Autodesk Inventor part; units mm, degrees
ref_plane "作業平面6" through (17, 0, 0) normal (1, 0, 0) x (0, 1, 0)
ref_plane "作業平面7" through (-17, 0, 0) normal (1, 0, 0) x (0, 1, 0)
ref_plane "作業平面8" through (0, 17, 0) normal (0, 1, 0) x (-1, 0, 0)
sketch "スケッチ1" plane through (0, 0, 0) normal (0, 0, 1) x (1, 0, 0)
  circle A0 centre (0, 0) radius 17
  circle A1 centre (0, 0) radius 11.5
  dimension "d0" = 34
  dimension "d1" = 23
extrude "押し出し1" add sketch "スケッチ1" against normal blind 40
sketch "スケッチ3" plane through (0, 0, 0) normal (0, 0, 1) x (1, 0, 0)
  circle A0 centre (0, 0) radius 15
  dimension "d8" = 30
extrude "押し出し3" cut sketch "スケッチ3" against normal blind 28
ref_plane "作業平面6" through (17, 0, 0) normal (1, 0, 0) x (0, 1, 0)
ref_plane "作業平面7" through (-17, 0, 0) normal (1, 0, 0) x (0, 1, 0)
sketch "スケッチ14" plane through (17, 0, 0) normal (1, 0, 0) x (0, 1, 0)
  point P0 (0, 0)
sketch "スケッチ15" plane through (17, 0, 0) normal (1, 0, 0) x (0, 1, 0)
  circle A0 centre (0, -5) radius 1.15
  point P0 (0, 0)
  dimension "d54" = 2.3
  dimension "d55" = 5
ref_plane "作業平面8" through (0, 17, 0) normal (0, 1, 0) x (-1, 0, 0)
ref_plane "作業平面9" through (0, -17, 0) normal (0, 1, 0) x (-1, 0, 0)
sketch "スケッチ16" plane through (0, 17, 0) normal (0, 1, 0) x (-1, 0, 0)
  circle A0 centre (0, -5) radius 1.15
  point P0 (0, 0)
  dimension "d58" = 2.3
  dimension "d59" = 5
extrude "押し出し13" cut sketch "スケッチ15" against normal through all
extrude "押し出し14" cut sketch "スケッチ16" against normal blind 5
sketch "スケッチ19" plane through (17, 0, 0) normal (1, 0, 0) x (0, 1, 0)
  circle A0 centre (0, -5) radius 2.1
  line L0 (17, 0) -> (-17, 0)
  point P0 (0, 0)
  dimension "d64" = 4.2
  dimension "d65" = 5
extrude "押し出し15" cut sketch "スケッチ19" against normal blind 1
sketch "スケッチ20" plane through (0, 17, 0) normal (0, 1, 0) x (-1, 0, 0)
  circle A0 centre (0, -5) radius 2.1
  line L0 (17, 0) -> (-17, 0)
  point P0 (0, 0)
  dimension "d68" = 4.2
  dimension "d69" = 5
extrude "押し出し16" cut sketch "スケッチ20" against normal blind 1
sketch "スケッチ21" plane through (-17, 0, 0) normal (1, 0, 0) x (0, 1, 0)
  circle A0 centre (0, -5) radius 2.1
  line L0 (17, 0) -> (-17, 0)
  point P0 (0, 0)
  dimension "d72" = 4.2
  dimension "d73" = 5
extrude "押し出し17" cut sketch "スケッチ21" along normal blind 1
sketch "スケッチ22" plane through (0, -17, 0) normal (0, 1, 0) x (-1, 0, 0)
  point P0 (0, 0)
sketch "スケッチ24" plane through (0, 0, -40) normal (0, 0, -1) x (-1, 0, 0)
  circle A0 centre (0, 0) radius 17
  circle A1 centre (0, 0) radius 13.4
  dimension "d80" = 26.8
  dimension "d83" = 34
extrude "押し出し19" cut sketch "スケッチ24" against normal blind 10
equation "\"BendRadius\" = Thickness"
equation "\"BendReliefWidth\" = Thickness"
equation "\"BendReliefDepth\" = 0.5 * Thickness"
equation "\"CornerReliefSize\" = 4 * Thickness"
equation "\"MinimumRemnant\" = 2 * Thickness"
equation "\"TransitionRadius\" = BendRadius"
equation "\"JacobiRadiusSize\" = BendRadius"
equation "\"GapSize\" = Thickness"
properties part number "B_pipe_adapter_1" material "ステンレス鋼 440C"
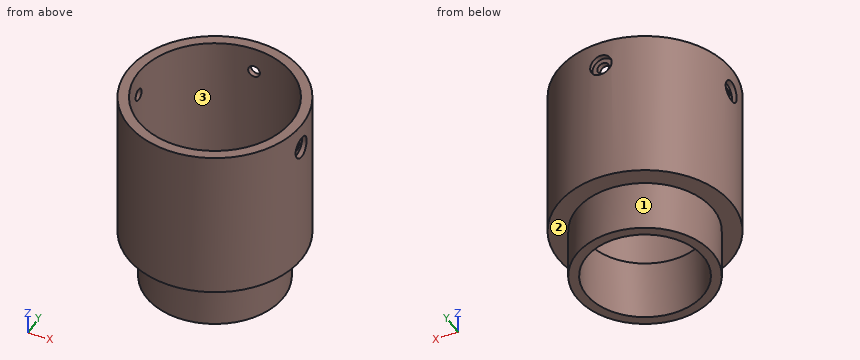
Here's how the part is built. I have some questions about the finished solid (model axes, mm). Face numbers are marked on the shaded views. Coordinates: 2 decimals unless noted, no trailing zeros. Loops run counter-clockwise (first coordinate to the right, second up) from the corner with the lowest first, then second, coordinate; pieces in that order, holes last. Notation, with made-up numbers: (88, 10.5) - (115, 10.5) arc R19 ccw to (115, 31.5) - close; hole circle Ø7 at (-30.5, 20.5). An arc over 180 degrees is marked (long way). Return JSON: item names as keys, results as strings. Group by question number.
Item 1: If we section it at B-B on y = 0: State how many separate pieces and enclosed holes the cut face has, and give its area (3 significant figures).
Item 2: If we section it at D-D on z = -5: Write out the boundary of the cut face in (x, y), and give its area (3 significant figures).
Item 3: If we section it at C-C on x = 4: Write out the boundary of the cut face in (y, z).
Item 4: I need wall thicknesses on line 1 (Y direction, x = 0, z = -31); line 2 (Z direction, x = 15.4, y = 0); line 3 (Z direction, x = 16.35, y = 0). Which ranges of each line are inside material? Lowest first, please. Write a range as from..to.
Item 5: Will these pins go through, and if not, where does the flat tip stop? P1, Ø2.5, axis at x = 0, z = -5, coming from the +Y side; P2, Ø2, axis at y = 11, z = -6.5, coming from the -X side; P3, Ø4, axis at y = 0, z = -5, coming from the -X side; P4, Ø10, axis at x = 2, z = -33.5, coming from the +Y side.
Item 6: We'd pull the mould along X, two halves only. Please class the marked faces 1, 2 and 3: +X half, -X half, draft (parallel to the pull), parting line (faces both ways), or undercut.
Item 7: If we section it at A-A on x = 0: Write out the boundary of the cut face in (y, z).
Calculated:
{
 "1": {"separate pieces": "4", "enclosed holes": "0", "area": "159 mm^2"},
 "2": {"outline": "(-16.87, -2.1) arc R17 ccw to (16.87, -2.1) - (16, -2.1) - (16, -1.15) - (14.96, -1.15) arc R15 cw to (-14.96, -1.15) - (-16, -1.15) - (-16, -2.1) - close; (-16.87, 2.1) - (-16, 2.1) - (-16, 1.15) - (-14.96, 1.15) arc R15 cw to (-1.15, 14.96) - (-1.15, 16) - (-2.1, 16) - (-2.1, 16.87) arc R17 ccw to start; (1.15, 14.96) arc R15 cw to (14.96, 1.15) - (16, 1.15) - (16, 2.1) - (16.87, 2.1) arc R17 ccw to (2.1, 16.87) - (2.1, 16) - (1.15, 16) - close", "area": "182 mm^2"},
 "3": {"outline": "(-16.52, -30) - (-12.79, -30) - (-12.79, -40) - (-10.78, -40) - (-10.78, -28) - (-14.46, -28) - (-14.46, 0) - (-16.52, 0) - close; (10.78, -40) - (12.79, -40) - (12.79, -30) - (16.52, -30) - (16.52, 0) - (14.46, 0) - (14.46, -28) - (10.78, -28) - close"},
 "4": {"line 1": "y = -13.4..-11.5, 11.5..13.4", "line 2": "z = -30..-6.15, -3.85..0", "line 3": "z = -30..-7.1, -2.9..0"},
 "5": {"P1": "stops at y = 16", "P2": "stops at x = -13.75", "P3": "stops at x = -16", "P4": "stops at y = 17"},
 "6": {"face 1": "parting line", "face 2": "draft", "face 3": "undercut"},
 "7": {"outline": "(-17, -30) - (-13.4, -30) - (-13.4, -40) - (-11.5, -40) - (-11.5, -28) - (-15, -28) - (-15, 0) - (-17, 0) - close; (11.5, -40) - (13.4, -40) - (13.4, -30) - (17, -30) - (17, -7.1) - (16, -7.1) - (16, -6.15) - (15, -6.15) - (15, -28) - (11.5, -28) - close; (15, -3.85) - (16, -3.85) - (16, -2.9) - (17, -2.9) - (17, 0) - (15, 0) - close"}
}
